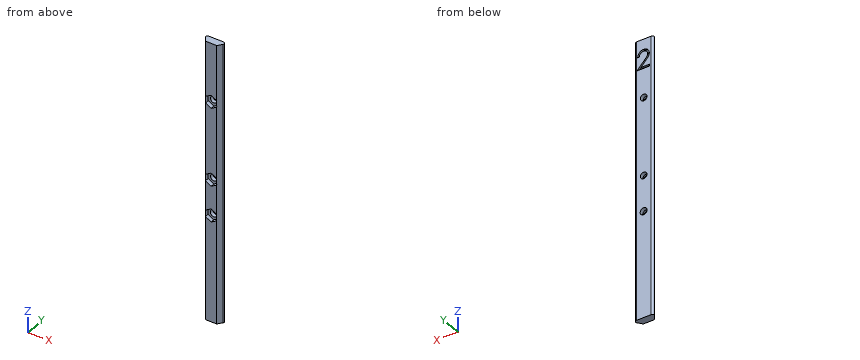
from build123d import *

# Parameters (mm, degrees)
BOSS_EXTRUDE1_DEPTH = 143
FILLET1_R           = 1
SKETCH2_R           = 1.8
CUT_EXTRUDE1_DEPTH  = 200
CUT_EXTRUDE2_DEPTH  = 2
CUT_EXTRUDE3_DEPTH  = 1
SKETCH5_R           = 1.7
CUT_EXTRUDE4_DEPTH  = 10
LPATTERN1_COUNT     = 2
LPATTERN1_PITCH     = 40
CUT_EXTRUDE5_DEPTH  = 2


with BuildPart() as part:
    # Sketch1 → Boss-Extrude1 (new body)
    with BuildSketch(Plane.XY):
        Polygon((0, 0), (5.8, 0), (8.7, 3.9), (-2.9, 3.9), align=None)
    extrude(amount=BOSS_EXTRUDE1_DEPTH)

    # Fillet1
    fillet1_edges = [part.edges().sort_by_distance(p)[0] for p in [
        (-2.9, 3.9, 71.5),
        (8.7, 3.9, 71.5),
    ]]
    fillet(fillet1_edges, radius=FILLET1_R)

    # Sketch2 → Cut-Extrude1 (cut)
    with BuildSketch(Plane.XZ):
        with Locations(Location((2.9, 54.6, 0), (0, 0, 270))):
            Circle(SKETCH2_R)
    extrude(amount=-CUT_EXTRUDE1_DEPTH, mode=Mode.SUBTRACT)

    # Sketch3 → Cut-Extrude2 (cut)
    with BuildSketch(Plane.XZ):
        Polygon((2.90000734, 57.948631561), (3.67e-06, 56.274322137), (-3.67e-06, 52.925690576), (2.89999266, 51.251368439), (5.79999633, 52.925677863), (5.80000367, 56.274309424), align=None)
    extrude(amount=-CUT_EXTRUDE2_DEPTH, mode=Mode.SUBTRACT)

    # Sketch4 → Cut-Extrude3 (cut)
    with BuildSketch(Plane(origin=(0, 3.9, 0), x_dir=(1, 0, 0), z_dir=(0, 1, 0))):
        with BuildLine():
            Line((5.122745858, -134.594230769), (5.977553551, -134.594230769))
            add(Edge.make_bspline(
                [(5.977553551, -134.594230769), (5.971983318, -134.707635673), (5.96104353, -134.930359885), (5.909790268, -135.255083464), (5.836521158, -135.565504079), (5.732681737, -135.858960447), (5.604449126, -136.138958148), (5.447455301, -136.401779138), (5.265047116, -136.650031883), (5.057559206, -136.879016136), (4.832415701, -137.088336373), (4.59096556, -137.271007952), (4.335690435, -137.423581719), (4.068804473, -137.551823488), (3.787221058, -137.647967628), (3.493631813, -137.719336337), (3.186709745, -137.762268246), (2.977595349, -137.766883522), (2.871243455, -137.769230769)],
                knots=[0, 0, 0, 0, 1.100776268, 2.161895295, 3.184016182, 4.190939212, 5.176500551, 6.166955529, 7.155448256, 8.160289653, 9.16017456, 10.133824356, 11.091467644, 12.04088621, 13.000931625, 13.972173743, 14.968683325, 16, 16, 16, 16], degree=3))
            add(Edge.make_bspline(
                [(2.871243455, -137.769230769), (2.766792917, -137.766805526), (2.561551342, -137.76204001), (2.26212941, -137.720499656), (1.976409076, -137.656842765), (1.707628406, -137.56251328), (1.453028956, -137.444150411), (1.215763088, -137.296950676), (0.990093468, -137.127879071), (0.787095567, -136.928450822), (0.600617505, -136.715660377), (0.43988469, -136.488401971), (0.301460326, -136.253409781), (0.188164307, -136.008848177), (0.102280887, -135.753920747), (0.038649503, -135.491071568), (0.002274366, -135.217267183), (-0.003277626, -135.031914725), (-0.006100295, -134.937680288)],
                knots=[0, 0, 0, 0, 1.111674182, 2.184400057, 3.212814286, 4.223731311, 5.211378316, 6.196328225, 7.191884489, 8.207283132, 9.220262353, 10.201199469, 11.166417575, 12.120932471, 13.06540007, 14.026332106, 14.996573967, 16, 16, 16, 16], degree=3))
            add(Edge.make_bspline(
                [(-0.006100295, -134.937680288), (-0.001492129, -134.805016596), (0.007643337, -134.54201727), (0.0857864, -134.155533128), (0.207837017, -133.781085653), (0.354773944, -133.479711723), (0.503045957, -133.236892134), (0.63652693, -133.036867771), (0.79367716, -132.821551985), (0.973154024, -132.590073288), (1.178048369, -132.345463088), (1.403037067, -132.082730681), (1.653930529, -131.806734169), (1.829867162, -131.618102024), (1.921033118, -131.520357572)],
                knots=[0, 0, 0, 0, 1.184416499, 2.348048165, 3.509039915, 4.696071444, 5.333504901, 6.05069495, 6.844171097, 7.714965912, 8.667477798, 9.695072654, 10.805644396, 12, 12, 12, 12], degree=3))
            Line((1.921033118, -131.520357572), (4.304191171, -128.976923077))
            Line((4.304191171, -128.976923077), (-0.12821568, -128.976923077))
            Line((-0.12821568, -128.976923077), (-0.12821568, -128))
            Line((-0.12821568, -128), (6.343899705, -128))
            Line((6.343899705, -128), (2.64990932, -131.94203726))
            add(Edge.make_bspline(
                [(2.64990932, -131.94203726), (2.559965489, -132.035916816), (2.387201798, -132.216240231), (2.142948702, -132.479586657), (1.923217267, -132.723609906), (1.727861736, -132.949391305), (1.55672137, -133.155650884), (1.410343741, -133.344005051), (1.288081888, -133.512837404), (1.158509801, -133.711174594), (1.034954218, -133.953619944), (0.926361503, -134.248410515), (0.860620951, -134.552545379), (0.85269448, -134.758008475), (0.848707397, -134.861358173)],
                knots=[0, 0, 0, 0, 1.329530082, 2.553755191, 3.672934919, 4.687409497, 5.60679272, 6.413407421, 7.126401618, 7.737995624, 8.834647426, 9.90044882, 10.943907757, 12, 12, 12, 12], degree=3))
            add(Edge.make_bspline(
                [(0.848707397, -134.861358173), (0.850419752, -134.926356875), (0.853794476, -135.054456835), (0.884142204, -135.242148032), (0.928729039, -135.423900083), (0.997451125, -135.597465755), (1.080018182, -135.766258747), (1.185503685, -135.925147228), (1.306045915, -136.079547323), (1.445868989, -136.224164782), (1.599368744, -136.356656831), (1.761555505, -136.474013435), (1.933140485, -136.572091957), (2.113408614, -136.652492299), (2.301855113, -136.715562491), (2.498845054, -136.759264755), (2.703833976, -136.786703519), (2.843806562, -136.790416014), (2.915128671, -136.792307692)],
                knots=[0, 0, 0, 0, 0.991504627, 1.954065223, 2.895985987, 3.842598665, 4.797835564, 5.759220273, 6.74786863, 7.784730864, 8.824135544, 9.839918996, 10.835834653, 11.835434876, 12.84861661, 13.863796685, 14.911511676, 16, 16, 16, 16], degree=3))
            add(Edge.make_bspline(
                [(2.915128671, -136.792307692), (2.989635464, -136.790439156), (3.135954505, -136.786769659), (3.350321609, -136.758957907), (3.556252164, -136.716838427), (3.750572839, -136.649784559), (3.937350419, -136.571306767), (4.111820115, -136.469691831), (4.278882998, -136.353581052), (4.435180219, -136.218203259), (4.577533213, -136.065382121), (4.707033005, -135.899039013), (4.816759463, -135.716225009), (4.914162533, -135.521326783), (4.988656651, -135.308989677), (5.052343784, -135.084406654), (5.098605194, -134.844373441), (5.11456532, -134.678996532), (5.122745858, -134.594230769)],
                knots=[0, 0, 0, 0, 1.031072318, 2.024855787, 2.988461151, 3.935103592, 4.865765533, 5.788564469, 6.724086513, 7.67908574, 8.64457978, 9.611397706, 10.591395687, 11.591555111, 12.622101007, 13.700900657, 14.821571223, 16, 16, 16, 16], degree=3))
        make_face()
    extrude(amount=-CUT_EXTRUDE3_DEPTH, mode=Mode.SUBTRACT)

    # Sketch5 → Cut-Extrude4 (cut)
    with BuildSketch(Plane(origin=(0, 3.9, 0), x_dir=(1, 0, 0), z_dir=(0, 1, 0))):
        with Locations(Location((2.9, -113, 0), (0, 0, 270))):
            Circle(SKETCH5_R)
    cut_extrude4 = extrude(amount=-CUT_EXTRUDE4_DEPTH, mode=Mode.SUBTRACT)

    # LPattern1: Cut-Extrude4 ×2
    with Locations(*[(0, 0, -i * LPATTERN1_PITCH) for i in range(1, LPATTERN1_COUNT)]):
        add(cut_extrude4, mode=Mode.SUBTRACT)

    # Sketch6 → Cut-Extrude5 (cut)
    with BuildSketch(Plane.XZ):
        Polygon((5.797077148, 114.679368135), (2.894163107, 116.348626474), (-0.002914041, 114.669258339), (0.002922852, 111.320631865), (2.905836893, 109.651373526), (5.802914041, 111.330741661), align=None)
        Polygon((5.797077148, 74.679368135), (2.894163107, 76.348626474), (-0.002914041, 74.669258339), (0.002922852, 71.320631865), (2.905836893, 69.651373526), (5.802914041, 71.330741661), align=None)
    extrude(amount=-CUT_EXTRUDE5_DEPTH, mode=Mode.SUBTRACT)


solid = part.part
Read the model definition and answer for the solid it produces. Units are mm, in the model's axes. Round coordinates to 2 decimals unless told otherwise and drop trailing zeros. Write each loop counter-clockwise with the first axis right and the second up, starting at its lowest first coordinate (ties: lowest second). Pieces come first, ordered by that corner, then holes.
Q1. Flat-ended cylindrical pins translate along their axes: P1, Ø3, axis at x = 3, z = 53.5, coming from the -Y side; P2, Ø1, axis at y = 0.5, z = 54, coming from the +X side; P3, Ø2, axis at y = 1.5, z = 54, coming from the -X side. Find the tip coordinate at first contact, or state that the pin passes through.
Values:
P1: stops at y = 2
P2: stops at x = 6.54
P3: stops at x = -1.83
Q2. Find section B-B on z = 61.5. Determine the outline of the cut face in (x, y), and give its area (3 significant figures).
Values:
outline: (-1.71, 2.3) - (0, 0) - (5.8, 0) - (7.51, 2.3) arc R1 ccw to (6.71, 3.9) - (-0.91, 3.9) arc R1 ccw to start
area: 32.2 mm2
Q3. Straight lines are drawn through the part: line 1 (Z direction, x = 3.25, y = 0.95); line 2 (X direction, y = 1.2, z = 136); line 3 (X direction, y = 2.7, z = 54.6). For each, find the intervals that lie inside material, in ascending order.
Values:
line 1: z = 0 to 51.45, 57.75 to 69.85, 76.14 to 109.85, 116.14 to 143
line 2: x = -0.89 to 6.69
line 3: x = -1.89 to 1.1, 4.7 to 7.69
Q4. Find section A-A on y = 1.35. Determine the outline of the cut face in (x, z), and give its area (3 significant figures).
Values:
outline: (-1, 0) - (6.8, 0) - (6.8, 143) - (-1, 143) - close; hole (0, 52.93) - (2.9, 51.25) - (5.8, 52.93) - (5.8, 56.27) - (2.9, 57.95) - (0, 56.27) - close; hole (0, 71.32) - (2.91, 69.65) - (5.8, 71.33) - (5.8, 74.68) - (2.89, 76.35) - (0, 74.67) - close; hole (0, 111.32) - (2.91, 109.65) - (5.8, 111.33) - (5.8, 114.68) - (2.89, 116.35) - (0, 114.67) - close
area: 1,030 mm2
